Could you check a few things on this model? Use its own coordinates, in mm. A direction names the side the tool comes from. Round coordinates to 2 decimals unless told otherwise and drop trailing zeros. Loops run counter-clockwise (first coordinate to the right, second up) from the corner with the lowest first, then second, coordinate; pieces in that order, holes last. Notation, with made-up numbers: (15.5, 13) - (53.5, 13) arc R9 ccw to (53.5, 22) - close; hole circle Ø7 at (41.5, 89). An arc over 180 degrees is marked (long way). Put each result on its own line as item: value. Start each with the question number.
from build123d import *

# Parameters (mm, degrees)
SKETCH3_R          = 1.706794341
CUT_EXTRUDE1_DEPTH = 10
SKETCH4_R          = 2.050203782
CUT_EXTRUDE2_DEPTH = 0.5
FILLET1_R          = 0.5
CHAMFER1_SIZE      = 0.1


with BuildPart() as part:
    # Sketch1 → Revolve1 (revolve)
    with BuildSketch(Plane.XY):
        Polygon((0, 0), (0, 2.58), (2.3, 3.196283143), (3.3, 3.196283143), (5, 2.793868124), (6.62, 2.793868124), (6.976131876, 3.15), (10.126131876, 3.15), (10.126131876, 3.3), (11, 3.3), (11, 2.15), (8.3, 2.15), (8.3, 0), align=None)
    revolve(axis=Axis((8.3, 0, 0), (-1, 0, 0)))

    # Sketch3 → Cut-Extrude1 (cut)
    with BuildSketch(Plane.ZY):
        with Locations(Location((0, 0, 0), (0, 0, 270))):
            Circle(SKETCH3_R)
    extrude(amount=-CUT_EXTRUDE1_DEPTH, mode=Mode.SUBTRACT)

    # Sketch4 → Cut-Extrude2 (cut)
    with BuildSketch(Plane.ZY):
        with Locations(Location((0, 0, 0), (0, 0, 270))):
            Circle(SKETCH4_R)
    extrude(amount=-CUT_EXTRUDE2_DEPTH, mode=Mode.SUBTRACT)

    # Fillet1
    fillet1_edges = [part.edges().sort_by_distance(p)[0] for p in [
        (0, -2.58, 0),
    ]]
    fillet(fillet1_edges, radius=FILLET1_R)

    # Chamfer1
    chamfer1_edges = [part.edges().sort_by_distance(p)[0] for p in [
        (11, -3.3, 0),
        (10.126131876, -3.15, 0),
    ]]
    chamfer(chamfer1_edges, length=CHAMFER1_SIZE)


solid = part.part
Item 1: Will these pins go through, and if not, where does the flat tip stop? P1, Ø1, axis at x = 9.5, z = -2.5, coming from the -Y side; P2, Ø1, axis at x = 5.5, y = -0.5, coming from the +Z side; P3, Ø2, axis at x = 8.5, z = -1.5, coming from the -Y side; P4, Ø1.3, axis at y = -0.5, z = -0.5, coming from the +X side.
Item 2: Suppose I cut it at B-B, the plane x = 6.5. List the corners of the cut face in (y, z) for me.
Item 3: On a 3-axis mill with a long thin cutter (end or side, diameter ignored), from which of +Z, -Z, +X, -X, +Y, -Y can I reach the whole of each face in a straight line? I mean faces 1 (the face through (2.81, 3.05, -0.96)), 2 (the face through (5.821, -0.606, 2.727)), 3 (the face through (4.35, -1.58, -0.65)), 4 (the face through (9.63, -2.15, -0.09)). Say none if no direction works.
Item 4: Suppose I cut it at A-A, the plane x = 9.75. List the corners of the cut face in (y, z) for me, then the cut area to 3 significant figures.
Item 5: I need wall thicknesses on line 1 (Y direction, x = 9.9, z = 0); line 2 (Y direction, x = 10.2, z = 0); line 3 (Z direction, x = 6.5, y = 0). Which ranges of each line are inside material? Lowest first, please. Write a range as from..to.
Item 6: Thinking about a two-plate mould opening in Z: for faces 5 (the face through (8.522, -2.5, 1.917)), 6 (the face through (0.246, -1.956, 0.616)), which applies, released by +Z, released by -Z, zero draft, split by the parting line, or undercut?
Numbers:
1. P1: y = -2.43
1. P2: z = 2.79
1. P3: y = -3.11
1. P4: through
2. outline: circle Ø5.59 at (0, 0); hole circle Ø3.41 at (0, 0)
3. face 1: -X
3. face 2: none
3. face 3: +X, -X
3. face 4: +X
4. outline: circle Ø6.3 at (0, 0); hole circle Ø4.3 at (0, 0)
4. area: 16.7 mm^2
5. line 1: -3.15..-2.15, 2.15..3.15
5. line 2: -3.3..-2.15, 2.15..3.3
5. line 3: -2.79..-1.71, 1.71..2.79
6. face 5: split by the parting line
6. face 6: undercut
